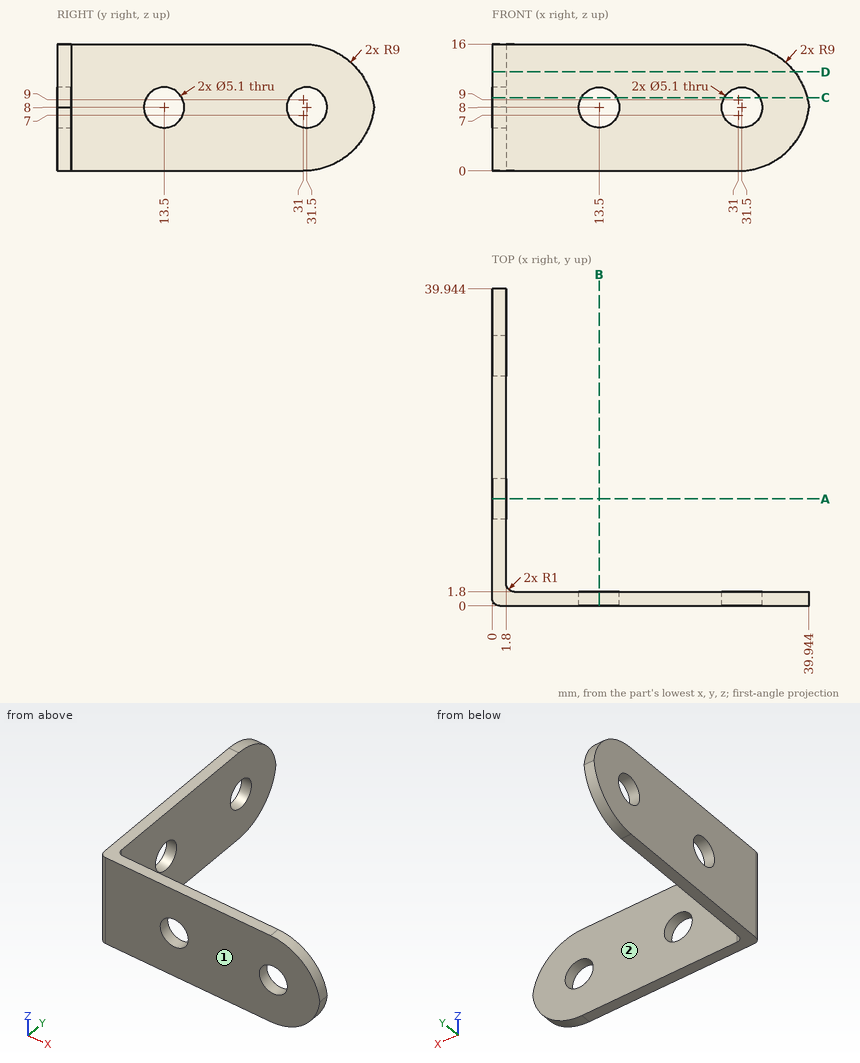
For this review, use the dimensioned drawing (mm, ordinates from the lowest corner) and the shaded views. A direction names the side the tool comes from. Coordinates: 2 decimals unless noted, no trailing zeros. Loops run counter-clockwise (first coordinate to the right, second up) from the corner with the lowest first, then second, coordinate; pieces in that order, holes last. Notation, with made-up numbers: (41, 58) -> (98, 58) arc R24 ccw to (98, 85) -> close; hole circle Ø9 at (39, -12). An arc over 180 degrees is marked (long way). Return JSON: item names as keys, results as strings. Group by question number.
(1) For pin 1 Ø5 at (y, z) = (17, 7.5) entering from +X; pin 2 Ø5 at (x, z) = (14.5, 8.5) entering from +Y, all flat-tipped, find the tip position at first contact; note any pin that passes through.
(2) To check wall thickness, follow L1, parallel to X at y = 1, z = 8; L2, parallel to Y at x = 37.5, z = 11. State the ranges of each line that lie inside material, in increasing order.
(3) Consider section A-A, the plane y = 13.5. Give the boundary of the cut face in (x, z).
(4) Consider section C-C, the plane z = 9.25. Give the boundary of the cut face in (x, y).
(5) Tool access review of the marked faces 1 and 2: name each direction out of +Z, -Z, +X, -X, +Y, -Y from which nothing blocks a thin tool from reaching the whole face with its end or side.
(6) Consider section D-D, the plane z = 12.5. Give the boundary of the cut face in (x, y).
Results below:
{
 "1": {"pin 1": "stops at x = 1.8", "pin 2": "stops at y = 1.8"},
 "2": {"L1": "x = 0 to 10.95, 16.05 to 28.95, 34.05 to 39.94", "L2": "y = 0 to 1.8"},
 "3": {"outline": "(0, 0) -> (1.8, 0) -> (1.8, 5.45) -> (0, 5.45) -> close; (0, 10.55) -> (1.8, 10.55) -> (1.8, 16) -> (0, 16) -> close"},
 "4": {"outline": "(0, 1) arc R1 ccw to (1, 0) -> (11.28, 0) -> (11.28, 1.8) -> (2.8, 1.8) arc R1 cw to (1.8, 2.8) -> (1.8, 11.28) -> (0, 11.28) -> close; (0, 15.72) -> (1.8, 15.72) -> (1.8, 29.28) -> (0, 29.28) -> close; (0, 33.72) -> (1.8, 33.72) -> (1.8, 39.71) -> (0, 39.71) -> close; (15.72, 0) -> (29.28, 0) -> (29.28, 1.8) -> (15.72, 1.8) -> close; (33.72, 0) -> (39.71, 0) -> (39.71, 1.8) -> (33.72, 1.8) -> close"},
 "5": {"face 1": "+Z, -Z, +X, -X, -Y", "face 2": "+Z, -Z, +X, +Y"},
 "6": {"outline": "(0, 1) arc R1 ccw to (1, 0) -> (38.12, 0) -> (38.12, 1.8) -> (2.8, 1.8) arc R1 cw to (1.8, 2.8) -> (1.8, 38.12) -> (0, 38.12) -> close"}
}
